Here's how the part is built. I have some questions about the finished solid (model axes, mm). Face numbers are marked on the shaded views. A direction names the side the tool comes from. Give positions to 0.01 mm unless a question says otherwise; leave off trailing zeros. One line per question, with ' | ' between items.
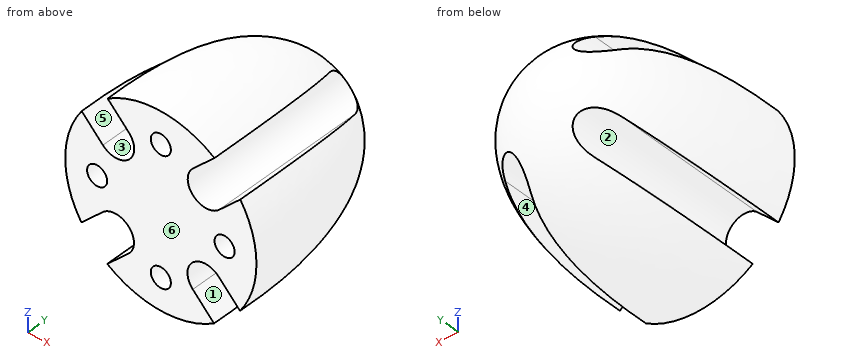
from build123d import *

# Parameters (mm, degrees)
SKETCH3_R          = 2.000000064
CUT_EXTRUDE1_DEPTH = 6.99999997
CUT_EXTRUDE3_REACH = 48.683


with BuildPart() as part:
    # Sketch1 → Revolve1 (revolve)
    with BuildSketch(Plane.XY):
        with BuildLine():
            Line((0, 0), (0, 38.1))
            add(Edge.make_bspline(
                [(0, 38.1), (19.753060043, 37.128354082), (19.05, 0)],
                knots=[0, 0, 0, 1, 1, 1], degree=2))
            Line((19.05, 0), (0, 0))
        make_face()
    revolve(axis=Axis((0, 0, 0), (0, 1, 0)))

    # Sketch3 → Cut-Extrude1 (cut)
    with BuildSketch(Plane.XZ):
        with Locations(Location((12.7, 0, 0), (0, 0, 270))):
            Circle(SKETCH3_R)
        with Locations(Location((-12.7, 0, 0), (0, 0, 270))):
            Circle(SKETCH3_R)
        with Locations(Location((0, 12.7, 0), (0, 0, 270))):
            Circle(SKETCH3_R)
        with Locations(Location((0, -12.7, 0), (0, 0, 270))):
            Circle(SKETCH3_R)
    extrude(amount=-CUT_EXTRUDE1_DEPTH, mode=Mode.SUBTRACT)

    # Sketch4 → Cut-Extrude3 (cut, up to next)
    with BuildSketch(Plane.XZ, mode=Mode.PRIVATE) as cut_extrude3_sk1:
        with BuildLine():
            Line((20.585051469, 15.321285367), (11.579529978, 6.366365899))
            ThreePointArc((11.579529978, 6.366365899), (6.416967921, 6.38091098), (6.431513003, 11.543473038))
            Line((6.431513003, 11.543473038), (15.437034493, 20.498392506))
            ThreePointArc((15.437034493, 20.498392506), (20.599596551, 20.483847424), (20.585051469, 15.321285367))
        make_face()
    cut_extrude3_tool1 = extrude(cut_extrude3_sk1.sketch, amount=-CUT_EXTRUDE3_REACH, mode=Mode.PRIVATE) & part.part
    # Sketch4 → Cut-Extrude3 (cut, up to next)
    with BuildSketch(Plane.XZ, mode=Mode.PRIVATE) as cut_extrude3_sk2:
        with BuildLine():
            Line((15.321285367, -20.585051469), (6.366365899, -11.579529978))
            ThreePointArc((6.366365899, -11.579529978), (6.38091098, -6.416967921), (11.543473038, -6.431513003))
            Line((11.543473038, -6.431513003), (20.498392506, -15.437034493))
            ThreePointArc((20.498392506, -15.437034493), (20.483847424, -20.599596551), (15.321285367, -20.585051469))
        make_face()
    cut_extrude3_tool2 = extrude(cut_extrude3_sk2.sketch, amount=-CUT_EXTRUDE3_REACH, mode=Mode.PRIVATE) & part.part
    # Sketch4 → Cut-Extrude3 (cut, up to next)
    with BuildSketch(Plane.XZ, mode=Mode.PRIVATE) as cut_extrude3_sk3:
        with BuildLine():
            Line((-20.585051469, -15.321285367), (-11.579529978, -6.366365899))
            ThreePointArc((-11.579529978, -6.366365899), (-6.416967921, -6.38091098), (-6.431513003, -11.543473038))
            Line((-6.431513003, -11.543473038), (-15.437034493, -20.498392506))
            ThreePointArc((-15.437034493, -20.498392506), (-20.599596551, -20.483847424), (-20.585051469, -15.321285367))
        make_face()
    cut_extrude3_tool3 = extrude(cut_extrude3_sk3.sketch, amount=-CUT_EXTRUDE3_REACH, mode=Mode.PRIVATE) & part.part
    # Sketch4 → Cut-Extrude3 (cut, up to next)
    with BuildSketch(Plane.XZ, mode=Mode.PRIVATE) as cut_extrude3_sk4:
        with BuildLine():
            Line((-15.321285367, 20.585051469), (-6.366365899, 11.579529978))
            ThreePointArc((-6.366365899, 11.579529978), (-6.38091098, 6.416967921), (-11.543473038, 6.431513003))
            Line((-11.543473038, 6.431513003), (-20.498392506, 15.437034493))
            ThreePointArc((-20.498392506, 15.437034493), (-20.483847424, 20.599596551), (-15.321285367, 20.585051469))
        make_face()
    cut_extrude3_tool4 = extrude(cut_extrude3_sk4.sketch, amount=-CUT_EXTRUDE3_REACH, mode=Mode.PRIVATE) & part.part
    add(cut_extrude3_tool1.solids().sort_by_distance((13.508282, 0, 13.432379))[0], mode=Mode.SUBTRACT)
    add(cut_extrude3_tool2.solids().sort_by_distance((13.432379, 0, -13.508282))[0], mode=Mode.SUBTRACT)
    add(cut_extrude3_tool3.solids().sort_by_distance((-13.508282, 0, -13.432379))[0], mode=Mode.SUBTRACT)
    add(cut_extrude3_tool4.solids().sort_by_distance((-13.432379, 0, 13.508282))[0], mode=Mode.SUBTRACT)


solid = part.part
1) Please list where these lines run through material, in increasing order: L1, parallel to X at y = 2, z = 0; L2, parallel to X at y = 13, z = 10; L3, parallel to Z at x = 7, y = 13.5.
Model answer:
L1: x = -19.07 to -14.7, -10.7 to 10.7, 14.7 to 19.07 | L2: x = -15.63 to -15.09, -5.44 to 5.51, 15.23 to 15.63 | L3: z = -17.13 to -12.22, -5.92 to 5.9, 12.11 to 17.13
2) I'm going to push flat-ended pins straight in: P1, Ø1.5, axis at x = 10, y = 22.5, coming from the +Z side; P2, Ø2, axis at x = 12, z = 4, coming from the +Y side; P3, Ø3.5, axis at x = 12.7, z = 0, coming from the -Y side; P4, Ø2, axis at x = 14.5, y = 31.5, coming from the +Z side. Where does each tip first touch, or does it pass through?
Model answer:
P1: stops at z = 5.75 | P2: stops at y = 32.63 | P3: stops at y = 7 | P4: passes through
3) I want a section at A-A (z = 8.5). State how many separate pieces and enclosed holes the cut face has, plus the area to 3 significant figures.
Model answer:
separate pieces: 3 | enclosed holes: 0 | area: 500 mm2
4) On a 3-axis mill with a long thin cutter (end or side, diameter ignored), from which of +Z, -Z, +X, -X, +Y, -Y can I reach the whole of each face in a straight line? I mean the marked faces 1 and 2. Say none if no direction works.
Model answer:
face 1: +X, +Y, -Y | face 2: +Y, -Y
5) Thinking about a two-plate mould opening in Z: for the marked faces 3, 4, 5 and 6, which applies, +Z half, -Z half, draft (parallel to the pull), parting line (faces both ways), or undercut?
Model answer:
face 3: undercut | face 4: -Z half | face 5: +Z half | face 6: draft
